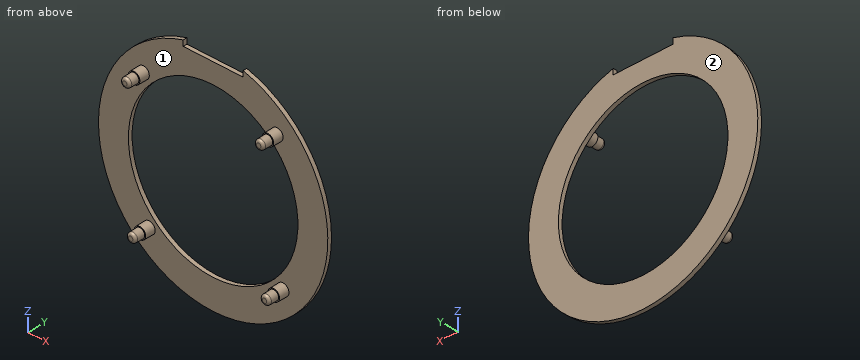
```python
from build123d import *

# Parameters (mm, degrees)
SKETCH1_R           = 11.5
SKETCH1_R_2         = 8.5
BOSS_EXTRUDE1_DEPTH = 0.4
SKETCH2_R           = 0.6
BOSS_EXTRUDE2_DEPTH = 1
SKETCH3_R           = 0.5
BOSS_EXTRUDE3_DEPTH = 1
CIRPATTERN1_COUNT   = 4
DRAFT1_ANGLE        = 1
FILLET1_R           = 0.25
CUT_EXTRUDE1_START  = -0.4
CUT_EXTRUDE1_DEPTH  = 0.4


with BuildPart() as part:
    # Sketch1 → Boss-Extrude1 (new body)
    with BuildSketch(Plane(origin=(0, 0, 0), x_dir=(1, 0, 0), z_dir=(0, 1, 0))):
        with Locations(Location((0, 1.53064501, 0), (0, 0, 270))):
            Circle(SKETCH1_R)
        with Locations(Location((0, 1.53064501, 0), (0, 0, 270))):
            Circle(SKETCH1_R_2, mode=Mode.SUBTRACT)
    extrude(amount=BOSS_EXTRUDE1_DEPTH)

    # Sketch2 → Boss-Extrude2 (add)
    with BuildSketch(Plane(origin=(0, 0, 0), x_dir=(1, 0, 0), z_dir=(0, 1, 0))):
        with Locations(Location((-7.0041347, -4.887461962, 0), (0, 0, 270))):
            Circle(SKETCH2_R)
    boss_extrude2 = extrude(amount=-BOSS_EXTRUDE2_DEPTH)

    # Sketch3 → Boss-Extrude3 (add)
    with BuildSketch(Plane.XZ.offset(1)):
        with Locations(Location((-7.0041347, 4.887461962, 0), (0, 0, 270))):
            Circle(SKETCH3_R)
    boss_extrude3 = extrude(amount=BOSS_EXTRUDE3_DEPTH)

    # CirPattern1: Boss-Extrude2, Boss-Extrude3 ×4 about axis
    cirpattern1_axis = Axis((0, 0, -1.53064501), (0, 1, 0))
    add([boss_extrude2.rotate(cirpattern1_axis, i * 360 / CIRPATTERN1_COUNT) for i in range(1, CIRPATTERN1_COUNT)])
    add([boss_extrude3.rotate(cirpattern1_axis, i * 360 / CIRPATTERN1_COUNT) for i in range(1, CIRPATTERN1_COUNT)])

    # Draft1
    draft1_faces = [part.faces().sort_by_distance(p)[0] for p in [
        (5.818106972, -0.5, 5.47348969),
        (6.918106972, -1.5, 5.47348969),
        (7.0041347, -0.5, -7.348751982),
        (7.0041347, -1.5, -8.448751982),
        (-5.818106972, -0.5, -8.53477971),
        (-6.918106972, -1.5, -8.53477971),
        (-7.0041347, -0.5, 4.287461962),
        (-7.0041347, -1.5, 5.387461962),
    ]]
    draft(draft1_faces, Plane(origin=(0, 0, -1.53064501), x_dir=(0, 0, -1), z_dir=(0, -1, 0)), DRAFT1_ANGLE)

    # Fillet1
    fillet1_edges = [part.edges().sort_by_distance(p)[0] for p in [
        (-7.0041347, -2, 5.352551832),
        (-6.883196842, -2, -8.53477971),
        (7.0041347, -2, -8.413841852),
        (6.883196842, -2, 5.47348969),
    ]]
    fillet(fillet1_edges, radius=FILLET1_R)

    # Sketch6 → Cut-Extrude1 (cut)
    with BuildSketch(Plane(origin=(0, 0.4, 0), x_dir=(1, 0, 0), z_dir=(0, 1, 0)).offset(CUT_EXTRUDE1_START)):
        with BuildLine():
            Line((3, -9), (-3, -9))
            Line((-3, -9), (-3, -9.571156646))
            ThreePointArc((-3, -9.571156646), (0, -9.96935499), (3, -9.571156646))
            Line((3, -9.571156646), (3, -9))
        make_face()
    extrude(amount=CUT_EXTRUDE1_DEPTH, mode=Mode.SUBTRACT)


solid = part.part
```
Could you check a few things on this model? Use its own coordinates, in mm. Face numbers are marked on the shaded views. Give positions to 0.01 mm unless a question says otherwise; leave off trailing zeros. Loops run counter-clockwise (first coordinate to the right, second up) from the corner with the lowest first, then second, coordinate; pieces in that order, holes last. Notation, with made-up numbers: (-8, 9.5) - (-1, 9.5) arc R11 cw to (-1, 15.5) - close; hole circle Ø4 at (73.25, 17). An arc over 180 degrees is marked (long way). Use one line per item in the form item = value.
1. I want a section at B-B (z = -1.5). Please give me the cut outline in (x, y), and give its area (3 significant figures).
Response values:
outline = (-11.5, 0) - (-8.5, 0) - (-8.5, 0.4) - (-11.5, 0.4) - close; (8.5, 0) - (11.5, 0) - (11.5, 0.4) - (8.5, 0.4) - close
area = 2.40 mm²
2. I need wall thicknesses on probe 1 along Y at (x, z) = (-8.25, -5.5); probe 2 along Z at (x, y) = (5, 0.3); probe 3 along Z at (x, y) = (-4.5, 0.1). Which ranges of each line are inside material? Lowest first, please.
Response values:
probe_1 = 0 to 0.4
probe_2 = -11.89 to -8.4, 5.34 to 8.83
probe_3 = -12.11 to -8.74, 5.68 to 9.05
3. I want a section at C-C (y = -0.4). Please give me the cut outline in (x, z).
Response values:
outline = circle Ø1.19 at (-7, 4.89); circle Ø1.19 at (-6.42, -8.53); circle Ø1.19 at (6.42, 5.47); circle Ø1.19 at (7, -7.95)
4. Thinking about a two-plate mould opening in Y: for the marked faces 1 and 2, which applies, released by +Y, released by -Y, zero draft, split by the parting line, or undercut?
Response values:
face_1 = released by -Y
face_2 = released by +Y
5. I'm going to push flat-ended pins straight in: pin 1 Ø1 at (x, y) = (-6.5, 0) entering from -Z; pin 2 Ø1 at (x, y) = (-3.5, 0) entering from -Z. Where does each tip first touch, or does it pass through?
Response values:
pin_1 = -11.34
pin_2 = -12.63
6. I want a section at A-A (x = 0). Please give me the cut outline in (y, z), and give its area (3 significant figures).
Response values:
outline = (0, -13.03) - (0.4, -13.03) - (0.4, -10.03) - (0, -10.03) - close; (0, 6.97) - (0.4, 6.97) - (0.4, 9) - (0, 9) - close
area = 2.01 mm²
